from build123d import *

# Parameters (mm, degrees)
F1_DEPTH = 1000


with BuildPart() as f1:
    # F0 (on Front) → F1 (new body)
    with BuildSketch(Plane.XZ):
        with BuildLine():
            Line((0, 50), (0, 0))
            Line((0, 0), (50, 0))
            Line((50, 0), (50, 5))
            ThreePointArc((50, 5), (36.819805, 36.819805), (5, 50))
            Line((5, 50), (0, 50))
        make_face()
    extrude(amount=-F1_DEPTH)


solid = f1.part
CAD build for the part. Positions are in the model's coordinates, mm. Coordinates: 2 decimals unless noted, no trailing zeros. Loops run counter-clockwise (first coordinate to the right, second up) from the corner with the lowest first, then second, coordinate; pieces in that order, holes last. Notation, with made-up numbers: (36.5, 50) - (48.5, 50) arc R22 cw to (48.5, 82) - close; hole circle Ø1 at (78, 74). An arc over 180 degrees is marked (long way). Write item = value, one per line. Start each with the question number.
Q1. Cut at A-A, the plane y = 258.5. List the corners of the cut face in (x, z).
Q2. Flat gauge pins, fed straight in: pin 1 Ø12 at (x, y) = (28.5, 324.5) entering from +Z; pin 2 Ø8 at (x, y) = (9.5, 221) entering from +Z. Where does each tip first touch, or does it go through?
Q3. Cut at B-B, the plane x = 41. List the corners of the cut face in (y, z).
Q4. Cut at C-C, the plane z = 39.5. List the corners of the cut face in (x, y), then the cut area to 3 significant figures.
Q5. Drill centre lines: L1, parallel to X at y = 785.5, z = 6.5 (3 decimals); L2, parallel to Z at x = 7, y = 691; L3, parallel to Z at x = 10.5, y = 426. Where is each one in solid material? Low to high.
Computed:
q1.outline = (0, 0) - (50, 0) - (50, 5) arc R45 ccw to (5, 50) - (0, 50) - close
q2.pin_1 = 46.46
q2.pin_2 = 50
q3.outline = (0, 0) - (1000, 0) - (1000, 32) - (0, 32) - close
q4.outline = (0, 0) - (33.89, 0) - (33.89, 1000) - (0, 1000) - close
q4.area = 33,900 mm²
q5.L1 = 0 to 49.975
q5.L2 = 0 to 49.96
q5.L3 = 0 to 49.66
